Build history of the part. All positions in model axes, mm. Face numbers are marked on the shaded views. A direction names the side the tool comes from. Round coordinates to 2 decimals unless told otherwise and drop trailing zeros. Loops run counter-clockwise (first coordinate to the right, second up) from the corner with the lowest first, then second, coordinate; pieces in that order, holes last. Notation, with made-up numbers: (-27, -27.75) - (-19, -27.75) arc R23 cw to (-19, -14.75) - close; hole circle Ø6 at (-10, 50.5). An arc over 180 degrees is marked (long way). Use one line per item in the form item = value. Start each with the question number.
Q1. 3-axis set-ups, long thin cutter, end or side, ignore diameter. For the marked faces 1 and 2: which of +Z, -Z, +X, -X, +Y, -Y reach the whole face in a straight line?
Q2. Pin check, flat tips, straight feed: pin 1 (6.5 mm diameter, centred on y = -40.5, z = 8.5, fed in from -X); pin 2 (10.5 mm diameter, centred on x = 30, y = -30, fed in from +Z); pin 3 (5 mm diameter, centred on y = -50, z = 10, fed in from +X); pin 4 (5 mm diameter, centred on y = -20, z = 10, fed in from -X). Stop position of each tip, or through.
Q3. Saw through at C-C (y = -20). Give the cut face in (x, z), then the cut area to 3 significant figures.
Q4. Saw through at A-A (x = 60). Give the cut face in (y, z), then the cut area to 3 significant figures.
Q5. Saw through at B-B (z = 2). Give the cut face in (x, y).
Q6. Saw through at D-D (x = 30). Give the cut face in (y, z), then the cut area to 3 significant figures.
Q7. Mould opens along X. For the marked faces 3, 4 and 5 say: released by +X, released by -X, zero draft, split by the parting line, or undercut.
Q8. Drill centre lines: line 1 (Y direction, x = 6.25, z = 10); line 2 (Y direction, x = 30, z = 7.5); line 3 (Z direction, x = 112, y = -50). Where is each one in solid material? Low to high.
```python
from build123d import *

# Parameters (mm, degrees)
SKETCH1_W           = 120
SKETCH1_H           = 60
BOSS_EXTRUDE1_DEPTH = 20
SKETCH2_R           = 4
SKETCH2_R_2         = 6
CUT_EXTRUDE1_DEPTH  = 20
SKETCH3_R           = 16
SKETCH3_R_2         = 4
CUT_EXTRUDE2_DEPTH  = 10
SKETCH4_R           = 3
CUT_EXTRUDE4_DEPTH  = 10
CUT_EXTRUDE5_START  = -10
SKETCH5_R           = 3
CUT_EXTRUDE5_DEPTH  = 10


with BuildPart() as part:
    # Sketch1 → Boss-Extrude1 (new body)
    with BuildSketch(Plane.XY):
        with Locations((60, -30)):
            Rectangle(SKETCH1_W, SKETCH1_H)
    extrude(amount=BOSS_EXTRUDE1_DEPTH)

    # Sketch2 → Cut-Extrude1 (cut)
    with BuildSketch(Plane.XY.offset(20)):
        with Locations((30, -30)):
            Circle(SKETCH2_R)
        with Locations((60, -30)):
            Circle(SKETCH2_R_2)
        with Locations((90, -30)):
            Circle(SKETCH2_R)
    extrude(amount=-CUT_EXTRUDE1_DEPTH, mode=Mode.SUBTRACT)

    # Sketch3 → Cut-Extrude2 (cut)
    # profile 1 of 2: a face of its own
    with BuildSketch(Plane.XY.offset(20)):
        with Locations((30, -30)):
            Circle(SKETCH3_R)
        with Locations((30, -30)):
            Circle(SKETCH3_R_2, mode=Mode.SUBTRACT)
    # profile 2 of 2: a face of its own
    with BuildSketch(Plane.XY.offset(20)):
        with Locations((90, -30)):
            Circle(SKETCH3_R)
        with Locations((90, -30)):
            Circle(SKETCH3_R_2, mode=Mode.SUBTRACT)
    extrude(amount=-CUT_EXTRUDE2_DEPTH, mode=Mode.SUBTRACT)

    # Sketch4 → Cut-Extrude4 (cut)
    with BuildSketch(Plane(origin=(120, 0, 0), x_dir=(0, 0, -1), z_dir=(1, 0, 0))):
        with Locations(Location((-10, -10, 0), (0, 0, 90))):
            Circle(SKETCH4_R)
        with Locations(Location((-10, -20, 0), (0, 0, 90))):
            Circle(SKETCH4_R)
        with Locations(Location((-10, -40, 0), (0, 0, 90))):
            Circle(SKETCH4_R)
        with Locations(Location((-10, -50, 0), (0, 0, 90))):
            Circle(SKETCH4_R)
    extrude(amount=-CUT_EXTRUDE4_DEPTH, mode=Mode.SUBTRACT)

    # Sketch5 → Cut-Extrude5 (cut)
    with BuildSketch(Plane.ZY.offset(CUT_EXTRUDE5_START)):
        with Locations(Location((10, -10, 0), (0, 0, 90))):
            Circle(SKETCH5_R)
        with Locations(Location((10, -20, 0), (0, 0, 90))):
            Circle(SKETCH5_R)
        with Locations(Location((10, -40, 0), (0, 0, 90))):
            Circle(SKETCH5_R)
        with Locations(Location((10, -50, 0), (0, 0, 90))):
            Circle(SKETCH5_R)
    extrude(amount=CUT_EXTRUDE5_DEPTH, mode=Mode.SUBTRACT)


solid = part.part
```
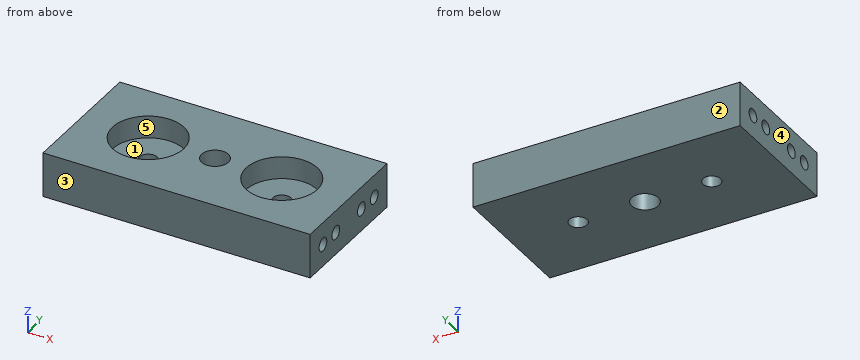
Report:
q1.face_1 = +Z
q1.face_2 = +Z, -Z, +X, -X, +Y
q2.pin_1 = 0
q2.pin_2 = 10
q2.pin_3 = 110
q2.pin_4 = 10
q3.outline = (0, 0) - (120, 0) - (120, 7) - (110, 7) - (110, 13) - (120, 13) - (120, 20) - (102.49, 20) - (102.49, 10) - (77.51, 10) - (77.51, 20) - (42.49, 20) - (42.49, 10) - (17.51, 10) - (17.51, 20) - (0, 20) - (0, 13) - (10, 13) - (10, 7) - (0, 7) - close
q3.area = 1,780 mm²
q4.outline = (-60, 0) - (-36, 0) - (-36, 20) - (-60, 20) - close; (-24, 0) - (0, 0) - (0, 20) - (-24, 20) - close
q4.area = 960 mm²
q5.outline = (0, -60) - (120, -60) - (120, 0) - (0, 0) - close; hole circle Ø8 at (30, -30); hole circle Ø12 at (60, -30); hole circle Ø8 at (90, -30)
q6.outline = (-60, 0) - (-34, 0) - (-34, 10) - (-46, 10) - (-46, 20) - (-60, 20) - close; (-26, 0) - (0, 0) - (0, 20) - (-14, 20) - (-14, 10) - (-26, 10) - close
q6.area = 800 mm²
q7.face_3 = zero draft
q7.face_4 = released by -X
q7.face_5 = undercut
q8.line_1 = -60 to -53, -47 to -43, -37 to -23, -17 to -13, -7 to 0
q8.line_2 = -60 to -34, -26 to 0
q8.line_3 = 0 to 7, 13 to 20
